```python
from build123d import *

# Parameters (mm, degrees)
SKETCH_R     = 1.6
PAD_DEPTH    = 4
SKETCH002_R  = 1.6
PAD001_DEPTH = 18.2
PAD002_DEPTH = 0.8


with BuildPart() as part:
    # Sketch → Pad (new body)
    with BuildSketch(Plane.XY):
        with BuildLine():
            ThreePointArc((-14.43353, 1.687235), (-20.512916, 1.781106), (-17.5, -3.5))
            Line((-17.5, -3.5), (-14.828962, -5.741267))
            ThreePointArc((-14.828962, -5.741267), (0.397332, -22.994737), (14.688532, -4.959109))
            Line((14.688532, -4.959109), (17.5, -3.5))
            ThreePointArc((17.5, -3.5), (20.51628, 1.775403), (14.439936, 1.698825))
            Line((13.896546, 1.698825), (14.439936, 1.698825))
            ThreePointArc((13.896546, 1.698825), (-0.005838, 13.999999), (-13.897958, 1.687235))
            Line((-14.43353, 1.687235), (-13.897958, 1.687235))
        make_face()
        with Locations((-17.5, 0)):
            Circle(SKETCH_R, mode=Mode.SUBTRACT)
        with Locations((17.5, 0)):
            Circle(SKETCH_R, mode=Mode.SUBTRACT)
    extrude(amount=PAD_DEPTH)

    # Sketch002 (on Face12 of Pad) → Pad001 (join)
    with BuildSketch(Plane.XY.offset(4)):
        with BuildLine():
            ThreePointArc((-14.43353, 1.687235), (-20.512916, 1.781106), (-17.5, -3.5))
            Line((-17.5, -3.5), (-14.828962, -5.741267))
            ThreePointArc((-14.828962, -5.741267), (0.397332, -22.994737), (14.688532, -4.959109))
            Line((14.688532, -4.959109), (17.5, -3.5))
            ThreePointArc((17.5, -3.5), (20.51628, 1.775403), (14.439936, 1.698825))
            Line((13.896546, 1.698825), (14.439936, 1.698825))
            ThreePointArc((12.792668, -5.6875), (13.846226, -2.069304), (13.896546, 1.698825))
            ThreePointArc((-12.792668, -5.6875), (0, -21), (12.792668, -5.6875))
            ThreePointArc((-13.897958, 1.687235), (-13.845362, -2.075078), (-12.792668, -5.6875))
            Line((-14.43353, 1.687235), (-13.897958, 1.687235))
        make_face()
        with Locations((-17.5, 0)):
            Circle(SKETCH002_R, mode=Mode.SUBTRACT)
        with Locations((17.5, 0)):
            Circle(SKETCH002_R, mode=Mode.SUBTRACT)
    extrude(amount=PAD001_DEPTH)

    # Sketch003 (on Face15 of Pad001) → Pad002 (join)
    with BuildSketch(Plane.XY.offset(22.2)):
        with BuildLine():
            Line((-17.5, -3.5), (-13.555442, -3.5))
            ThreePointArc((-13.555442, -3.5), (-13.21938, -4.609555), (-12.792668, -5.6875))
            ThreePointArc((-12.792668, -5.6875), (0, -21), (12.792668, -5.6875))
            ThreePointArc((12.792668, -5.6875), (13.21938, -4.609555), (13.555442, -3.5))
            Line((17.5, -3.5), (13.555442, -3.5))
            Line((17.5, -3.5), (14.688532, -4.959109))
            ThreePointArc((-14.828962, -5.741267), (0.397332, -22.994737), (14.688532, -4.959109))
            Line((-17.5, -3.5), (-14.828962, -5.741267))
        make_face()
    extrude(amount=PAD002_DEPTH)


solid = part.part
```
Build history of the part. All positions in model axes, mm. A direction names the side the tool comes from. Give positions to 0.01 mm unless a question says otherwise; leave off trailing zeros. Loops run counter-clockwise (first coordinate to the right, second up) from the corner with the lowest first, then second, coordinate; pieces in that order, holes last.
1) Band-saw the part on B-B on y = -8. List the corners of the cut face in (x, z).
Values follow:
outline: (-15, 0) - (15, 0) - (15, 23) - (13, 23) - (13, 4) - (-13, 4) - (-13, 23) - (-15, 23) - close
2) 3-axis set-ups, long thin cutter, end or side, ignore diameter. For faces 4 (the face through (16, -1, 22.2)), 5 (the face through (-13.853, -2.023, 12.973)), 6 (the face through (-19.1, 0.07, 10.94)): which of +Z, -Z, +X, -X, +Y, -Y reach the whole face in a straight line?
Values follow:
face 4: +Z, +X, -X, +Y
face 5: +Z
face 6: +Z, -Z
3) Drop flat-ended pins along their axis: P1, Ø1, axis at x = 0.5, z = 9.5, coming from the -Y side; P2, Ø0.6, axis at x = -14, z = 13.5, coming from the +Y side; P3, Ø4, axis at y = -18.5, z = 6.5, coming from the -X side; P4, Ø3, axis at x = 11.5, y = 5.5, coming from the +Z side. Give the stop position or say it passes through.
Values follow:
P1: stops at y = -23
P2: stops at y = 1.69
P3: stops at x = -12.36
P4: stops at z = 4
4) Band-saw the part on C-C on x = 0. List the corners of the cut face in (y, z), then the cut area to 3 significant figures.
Values follow:
outline: (-23, 0) - (14, 0) - (14, 4) - (-21, 4) - (-21, 23) - (-23, 23) - close
area: 186 mm2
5) Band-saw the part on D-D on x = 7.5. List the corners of the cut face in (y, z), then the cut area to 3 significant figures.
Values follow:
outline: (-20.99, 0) - (11.82, 0) - (11.82, 4) - (-18.62, 4) - (-18.62, 23) - (-20.99, 23) - close
area: 176 mm2
6) Band-saw the part on A-A on z = 13.25. List the corners of the cut face in (x, y), then the cut area to 3 significant figures.
Values follow:
outline: (-17.5, -3.5) - (-14.83, -5.74) arc R15 ccw (long way) to (14.69, -4.96) - (17.5, -3.5) arc R3.5 ccw (long way) to (14.44, 1.7) - (13.9, 1.7) arc R14 cw to (12.79, -5.69) arc R13 cw (long way) to (-12.79, -5.69) arc R14 cw to (-13.9, 1.69) - (-14.43, 1.69) arc R3.5 ccw (long way) to start; hole circle Ø3.2 at (-17.5, 0); hole circle Ø3.2 at (17.5, 0)
area: 177 mm2
7) Two-plate mould, pull along Y, no slides. Class faces 1 (the face through (13.84, -2.12, 12.97)), 2 (the face through (0.08, -21.15, 23)), 3 (the face through (-20.46, 1.87, 10.94)): released by +Y, released by -Y, zero draft, split by the parting line, or undercut.
Values follow:
face 1: undercut
face 2: zero draft
face 3: split by the parting line
8) Probe line 1 along X through (y, z) = (-8, 14.5); line 2 along Y through (x, z) = (17.5, 8); line 3 along X through (y, z) = (-1, 20). List the from-to ranges inside material, lowest first.
Values follow:
line 1: x = -15 to -13, 13 to 15
line 2: y = -3.5 to -1.6, 1.6 to 3.5
line 3: x = -20.85 to -18.75, -16.25 to -13.96, 13.96 to 16.25, 18.75 to 20.85
